Source: CAD feature listing. Evaluate the final solid. Frame: model axes, mm. A direction names the side the tool comes from. Give positions to 0.01 mm unless a question says otherwise; leave off trailing zeros. Loops run counter-clockwise (first coordinate to the right, second up) from the corner with the lowest first, then second, coordinate; pieces in that order, holes last.
```python
from build123d import *

# Parameters (mm, degrees)
F0_W     = 15.875
F0_H     = 12.7
F1_DEPTH = 12.7
F3_DEPTH = 12.7


with BuildPart() as f1:
    # F0 (on Top) → F1 (new body)
    with BuildSketch(Plane.XY):
        with Locations((23.8125, -19.05)):
            Rectangle(F0_W, F0_H)
        with BuildLine():
            ThreePointArc((31.75, 12.7), (44.45, 0), (31.75, -12.7))
            Line((31.75, -12.7), (31.75, -25.4))
            ThreePointArc((31.75, -25.4), (57.15, 0), (31.75, 25.4))
            Line((31.75, 25.4), (0, 25.4))
            Line((0, 25.4), (-31.75, 25.4))
            ThreePointArc((-31.75, 25.4), (-57.15, 0), (-31.75, -25.4))
            Line((-31.75, -25.4), (-15.875, -25.4))
            Line((-15.875, -25.4), (-15.875, -12.7))
            Line((-15.875, -12.7), (-31.75, -12.7))
            ThreePointArc((-31.75, -12.7), (-44.45, 0), (-31.75, 12.7))
            Line((-31.75, 12.7), (0, 12.7))
            Line((0, 12.7), (31.75, 12.7))
        make_face()
    extrude(amount=F1_DEPTH)

    # F2 (on face) → F3 (join)
    with BuildSketch(Plane.XZ.offset(-12.7)):
        with BuildLine():
            Line((14.2875, 25.4), (7.9375, 25.4))
            ThreePointArc((7.9375, 25.4), (0, 17.4625), (-7.9375, 25.4))
            Line((-7.9375, 25.4), (-14.2875, 25.4))
            Line((-14.2875, 25.4), (-14.2875, 12.7))
            Line((-14.2875, 12.7), (14.2875, 12.7))
            Line((14.2875, 12.7), (14.2875, 25.4))
        make_face()
        with BuildLine():
            ThreePointArc((-7.9375, 25.4), (0, 33.3375), (7.9375, 25.4))
            Line((7.9375, 25.4), (14.2875, 25.4))
            ThreePointArc((14.2875, 25.4), (0, 39.6875), (-14.2875, 25.4))
            Line((-14.2875, 25.4), (-7.9375, 25.4))
        make_face()
    extrude(amount=-F3_DEPTH)


solid = f1.part
```
(1) First-contact query: pin 1 (8 mm diameter, centred on y = -0.5, z = 4.5, fed in from +X); pin 2 (13 mm diameter, centred on x = -26, y = -1, fed in from +Z); pin 3 (4 mm diameter, centred on y = -18.5, z = 8.5, fed in from -X); pin 4 (6.5 mm diameter, centred on y = 19, z = 16.5, fed in from +X). Flat tips, straight axial feed; report the tip coordinate or a pass-through.
A:
pin 1: stops at x = 57.15
pin 2: passes through
pin 3: stops at x = -51.06
pin 4: stops at x = 14.29
(2) Ray query, line 1 along Z through (x, y) = (0, 15.5); line 2 along X through (y, z) = (21, 25); line 3 along Y through (x, z) = (-29, 2). Return the intervals inside material, ascending.
A:
line 1: z = 0 to 17.46, 33.34 to 39.69
line 2: x = -14.29 to -7.93, 7.93 to 14.29
line 3: y = -25.4 to -12.7, 12.7 to 25.4
(3) Section B-B, the plane y = 0. Return the cut outline in (x, z).
A:
outline: (-57.15, 0) - (-44.45, 0) - (-44.45, 12.7) - (-57.15, 12.7) - close; (44.45, 0) - (57.15, 0) - (57.15, 12.7) - (44.45, 12.7) - close
(4) Reachability of faces 4 (the flat face through (14.288, 19, 19)), 5 (the flat face through (-46, 0, 12.7)), 6 (the flat face through (-1, 17, 0)), 7 (the flat face through (24, -12.7, 6)), 8 (the flat face through (-15.875, -19, 6)) from +Z, -Z, +X, -X, +Y, -Y: full face, straight path, thin tool, end or side. Return the list, or none.
A:
face 4: +Z, +X, +Y, -Y
face 5: +Z, -X, +Y, -Y
face 6: -Z, +X, -X, +Y, -Y
face 7: +Z, -Z
face 8: +Z, -Z, -Y
(5) Section C-C, the plane z = 6. Return the cut outline in (x, y) (3 decimals).
A:
outline: (-31.75, -25.4) - (-15.875, -25.4) - (-15.875, -12.7) - (-31.75, -12.7) arc R12.7 cw to (-31.75, 12.7) - (31.75, 12.7) arc R12.7 cw to (31.75, -12.7) - (15.875, -12.7) - (15.875, -25.4) - (31.75, -25.4) arc R25.4 ccw to (31.75, 25.4) - (-31.75, 25.4) arc R25.4 ccw to start
(6) Mould query, pull axis Y, two halves, no side actions, for faces 1 (the flat face through (15.875, -19, 6)), 2 (the flat face through (-24, -25.4, 6)), 3 (the cylindrical face through (44.447, 0.279, 6.261)). Classes: pulls with the +Y half, pulls with the -Y half, needs draft (parallel to the pull), parting line crosses it, or undercut.
A:
face 1: needs draft
face 2: pulls with the -Y half
face 3: undercut
(7) Section D-D, the plane z = 34.5. Return the cut outline in (x, y), then the cut area to 3 significant figures.
A:
outline: (-11.01, 12.7) - (11.01, 12.7) - (11.01, 25.4) - (-11.01, 25.4) - close
area: 280 mm2
(8) Section A-A, the plane x = 28. Return the cut outline in (y, z), then the cut area to 3 significant figures.
A:
outline: (-25.4, 0) - (-12.7, 0) - (-12.7, 12.7) - (-25.4, 12.7) - close; (12.7, 0) - (25.4, 0) - (25.4, 12.7) - (12.7, 12.7) - close
area: 323 mm2
